Autodesk Inventor part; units mm, degrees
ref_plane "YZ Plane" through (0, 0, 0) normal (1, 0, 0) x (0, 1, 0)
ref_plane "XZ Plane" through (0, 0, 0) normal (0, 1, 0) x (-1, 0, 0)
ref_plane "XY Plane" through (0, 0, 0) normal (0, 0, 1) x (1, 0, 0)
sketch "Boceto1" plane through (0, 0, 0) normal (0, 0, 1) x (1, 0, 0)
  line L0 (206, -30) -> (206, 220)
  line L1 (0, 220) -> (206, 220)
  line L2 (0, -30) -> (0, 220)
  line L3 (206, -30) -> (0, -30)
  line L4 (206, -30) -> (206, -5)
  line L5 (206, -5) -> (203, -5)
  line L6 (203, -5) -> (203, 20)
  line L7 (203, 20) -> (206, 20)
  line L8 (206, 20) -> (206, 45)
  line L9 (206, 45) -> (203, 45)
  line L10 (203, 45) -> (203, 70)
  line L11 (203, 70) -> (206, 70)
  line L12 (206, 70) -> (206, 95)
  line L13 (206, 95) -> (203, 95)
  line L14 (203, 95) -> (203, 120)
  line L15 (203, 120) -> (206, 120)
  line L16 (206, 120) -> (206, 145)
  line L17 (206, 145) -> (203, 145)
  line L18 (203, 145) -> (203, 170)
  line L19 (203, 170) -> (206, 170)
  line L20 (203, 220) -> (206, 220)
  line L21 (206, 195) -> (203, 195)
  line L22 (203, 195) -> (203, 220)
  line L23 (206, 170) -> (206, 195)
  line L24 (203, 170) -> (206, 170)
  line L25 (0, 220) -> (0, 195)
  line L26 (0, 195) -> (3, 195)
  line L27 (3, 195) -> (3, 170)
  line L28 (3, 170) -> (0, 170)
  line L29 (0, 170) -> (0, 145)
  line L30 (0, 145) -> (3, 145)
  line L31 (3, 145) -> (3, 120)
  line L32 (3, 120) -> (0, 120)
  line L33 (3, 20) -> (0, 20)
  line L34 (0, 45) -> (3, 45)
  line L35 (3, 45) -> (3, 20)
  line L36 (0, 70) -> (0, 45)
  line L37 (3, 70) -> (0, 70)
  line L38 (3, 95) -> (3, 70)
  line L39 (0, 95) -> (3, 95)
  line L40 (0, 120) -> (0, 95)
  line L41 (3, 20) -> (0, 20)
  line L42 (0, 20) -> (0, -5)
  line L43 (0, -5) -> (3, -5)
  line L44 (3, -5) -> (3, -30)
  line L45 (3, -30) -> (0, -30)
  line L46 (203, 220) -> (206, 220)
  line L47 (203, 220) -> (206, 220)
  line L48 (206, 220) -> (206, 245)
  line L49 (206, 245) -> (203, 245)
  line L50 (203, 245) -> (203, 270)
  line L51 (203, 270) -> (206, 270)
  line L52 (0, 220) -> (3, 220)
  line L53 (0, 220) -> (3, 220)
  line L54 (3, 220) -> (3, 245)
  line L55 (3, 245) -> (0, 245)
  line L56 (0, 245) -> (0, 270)
  line L57 (0, 270) -> (3, 270)
  line L58 (206, 270) -> (0, 270)
  point P0 (0, 0)
  dimension "d78" = 3
  dimension "d88" = 3
  dimension "Lengueta" = 25
  dimension "espesor" = 3
  dimension "d2" = 25
  dimension "d3" = 3
  dimension "d4" = 25
  dimension "d5" = 90
  dimension "d6" = 3
  dimension "d7" = 25
  dimension "d8" = 3
  dimension "d9" = 25
  dimension "d10" = 3
  dimension "d11" = 25
  dimension "d12" = 3
  dimension "d13" = 25
  dimension "d14" = 90
  dimension "d15" = 3
  dimension "d16" = 25
  dimension "d17" = 3
  dimension "d18" = 3
  dimension "d19" = 25
  dimension "d20" = 90
  dimension "d21" = 3
  dimension "d22" = 25
  dimension "d23" = 3
  dimension "d26" = 25
  dimension "d27" = 3
  dimension "d28" = 25
  dimension "d29" = 3
  dimension "d30" = 25
  dimension "d31" = 90
  dimension "d32" = 3
  dimension "d33" = 25
  dimension "d34" = 3
  dimension "d35" = 25
  dimension "d36" = 3
  dimension "d37" = 25
  dimension "d38" = 3
  dimension "d39" = 25
  dimension "d40" = 90
  dimension "d41" = 3
  dimension "d42" = 25
  dimension "d43" = 3
  dimension "d44" = 3
  dimension "d45" = 25
  dimension "d46" = 90
  dimension "d47" = 3
  dimension "d48" = 25
  dimension "d49" = 3
  dimension "d71" = 3
  dimension "d72" = 3
  dimension "d73" = 25
  dimension "d74" = 90
  dimension "d75" = 3
  dimension "d76" = 25
  dimension "d77" = 3
  dimension "d81" = 3
  dimension "d82" = 3
  dimension "d83" = 25
  dimension "d84" = 90
  dimension "d85" = 3
  dimension "d86" = 25
  dimension "d87" = 3
extrude "Extrusión1" add sketch "Boceto1" against normal blind 3 contours L3 L44 L43 L2 L33 L35 L34 L37 L38 L39 L32 L31 L30 L28 L27 L26 L1 L22 L21 L0 L19 L18 L17 L15 L14 L13 L11 L10 L9 L7 L6 L5
sketch "Boceto2" plane through (0, 0, 0) normal (0, 0, 1) x (1, 0, 0)
  circle A0 centre (53, -15) radius 1.75
  circle A1 centre (153, -15) radius 1.75
  point P0 (0, 0)
extrude "Extrusión2" cut sketch "Boceto2" against normal blind 3
sketch "Boceto3" plane through (0, 0, 0) normal (0, 0, 1) x (1, 0, 0)
  circle A0 centre (53, 208) radius 2.1
  circle A1 centre (53, 208) radius 1.5
  circle A2 centre (153, 208) radius 2.1
  point P0 (0, 0)
  dimension "d56" = 3
hole "Agujero1" at (53, 208, 0) at (153, 208, 0) direction (0, 0, -1) diameter 3 depth 4
sketch "Boceto4" plane through (0, 0, 0) normal (0, 0, 1) x (1, 0, 0)
  circle A0 centre (53, 85) radius 2.1
  circle A1 centre (153, 85) radius 2.1
  point P0 (0, 0)
hole "Agujero2" at (153, 85, 0) at (53, 85, 0) direction (0, 0, -1) diameter 3 depth 4
sketch "Boceto5" plane through (0, 0, -3) normal (0, 0, -1) x (-1, 0, 0)
  point P0 (0, 0)
sketch "Boceto6" plane through (0, 0, 0) normal (0, 0, 1) x (1, 0, 0)
  circle A0 centre (53, 85) radius 1.5
  circle A1 centre (153, 85) radius 1.5
  circle A2 centre (153, 208) radius 1.5
  circle A3 centre (53, 208) radius 1.5
  circle A4 centre (53, -15) radius 1.75
  circle A5 centre (153, -15) radius 1.75
  line L0 (203, 20) -> (206, 20)
  line L1 (206, 20) -> (206, 45)
  line L2 (206, 45) -> (203, 45)
  line L3 (203, 45) -> (203, 70)
  line L4 (203, 70) -> (206, 70)
  line L5 (206, 70) -> (206, 95)
  line L6 (206, 95) -> (203, 95)
  line L7 (203, 95) -> (203, 120)
  line L8 (203, 120) -> (206, 120)
  line L9 (206, 120) -> (206, 145)
  line L10 (206, 145) -> (203, 145)
  line L11 (203, 145) -> (203, 170)
  line L12 (203, 170) -> (206, 170)
  line L13 (206, 170) -> (206, 195)
  line L14 (206, 195) -> (203, 195)
  line L15 (203, 195) -> (203, 220)
  line L16 (203, 220) -> (0, 220)
  line L17 (0, 220) -> (0, 195)
  line L18 (0, 195) -> (3, 195)
  line L19 (3, 195) -> (3, 170)
  line L20 (3, 170) -> (0, 170)
  line L21 (0, 170) -> (0, 145)
  line L22 (0, 145) -> (3, 145)
  line L23 (3, 145) -> (3, 120)
  line L24 (3, 120) -> (0, 120)
  line L25 (0, 120) -> (0, 95)
  line L26 (0, 95) -> (3, 95)
  line L27 (3, 95) -> (3, 70)
  line L28 (3, 70) -> (0, 70)
  line L29 (0, 70) -> (0, 45)
  line L30 (0, 45) -> (3, 45)
  line L31 (3, 45) -> (3, 20)
  line L32 (3, 20) -> (0, 20)
  line L33 (0, 20) -> (0, -5)
  line L34 (0, -5) -> (3, -5)
  line L35 (3, -5) -> (3, -30)
  line L36 (3, -30) -> (206, -30)
  line L37 (206, -30) -> (206, -5)
  line L38 (206, -5) -> (203, -5)
  line L39 (203, -5) -> (203, 20)
  line L40 (153, 85) -> (153, 208)
  line L41 (150.5, 161.5) -> (155.5, 161.5)
  line L42 (155.5, 161.5) -> (155.5, 131.5)
  line L43 (155.5, 131.5) -> (150.5, 131.5)
  line L44 (150.5, 131.5) -> (150.5, 161.5)
  line L45 (150.5, 161.5) -> (155.5, 131.5) construction
  line L46 (155.5, 161.5) -> (150.5, 131.5) construction
  line L47 (53, 85) -> (53, 208)
  line L48 (50.5, 161.5) -> (55.5, 161.5)
  line L49 (55.5, 161.5) -> (55.5, 131.5)
  line L50 (55.5, 131.5) -> (50.5, 131.5)
  line L51 (50.5, 131.5) -> (50.5, 161.5)
  line L52 (50.5, 161.5) -> (55.5, 131.5) construction
  line L53 (55.5, 161.5) -> (50.5, 131.5) construction
  line L54 (53, -15) -> (53, 85)
  line L55 (50.5, 50) -> (55.5, 50)
  line L56 (55.5, 50) -> (55.5, 20)
  line L57 (55.5, 20) -> (50.5, 20)
  line L58 (50.5, 20) -> (50.5, 50)
  line L59 (50.5, 50) -> (55.5, 20) construction
  line L60 (55.5, 50) -> (50.5, 20) construction
  line L61 (150.5, 50) -> (155.5, 50)
  line L62 (155.5, 50) -> (155.5, 20)
  line L63 (155.5, 20) -> (150.5, 20)
  line L64 (150.5, 20) -> (150.5, 50)
  line L65 (150.5, 50) -> (155.5, 20) construction
  line L66 (155.5, 50) -> (150.5, 20) construction
  point P0 (0, 0)
  point P1 (153, 146.5)
  point P2 (53, 146.5)
  point P3 (53, 35)
  point P4 (153, 35)
  dimension "d93" = 5
  dimension "d94" = 30
  dimension "d95" = 5
  dimension "d96" = 30
  dimension "d99" = 5
  dimension "d100" = 30
  dimension "d101" = 5
  dimension "d102" = 30
extrude "Extrusión3" cut sketch "Boceto6" against normal blind 3 contours L55 L56 L57 L54 | L54 L57 L58 L55 | L50 L51 L48 L47 | L47 L48 L49 L50 | L43 L44 L41 L40 | L40 L41 L42 L43 | L61 L62 L63 L64
sketch "Boceto7" plane through (0, 0, 0) normal (0, 0, 1) x (1, 0, 0)
  line L0 (3, 95.5) -> (60.5, 95.5)
  line L1 (60.5, 95.5) -> (60.5, 98.5)
  line L2 (60.5, 98.5) -> (3, 98.5)
  line L3 (3, 98.5) -> (3, 121)
  line L4 (3, 121) -> (60.5, 121)
  line L5 (60.5, 121) -> (60.5, 124)
  line L6 (60.5, 124) -> (3, 124)
  line L7 (3, 124) -> (3, 128)
  arc A0 (10.873, 129) -> (3, 128) centre (7, 128) ccw
  arc A1 (10.873, 129) -> (14.746, 126) centre (14.746, 130) ccw
  line L8 (14.746, 126) -> (57.754, 126)
  arc A2 (57.754, 126) -> (61.627, 129) centre (57.754, 130) ccw
  arc A3 (69.5, 128) -> (61.627, 129) centre (65.5, 128) ccw
  line L9 (69.5, 128) -> (69.5, 91.5)
  arc A4 (61.627, 90.5) -> (69.5, 91.5) centre (65.5, 91.5) ccw
  arc A5 (61.627, 90.5) -> (57.754, 93.5) centre (57.754, 89.5) ccw
  line L10 (57.754, 93.5) -> (14.746, 93.5)
  arc A6 (14.746, 93.5) -> (10.873, 90.5) centre (14.746, 89.5) ccw
  arc A7 (3, 91.5) -> (10.873, 90.5) centre (7, 91.5) ccw
  line L11 (3, 91.5) -> (3, 95.5)
  line L12 (66.1403, 93.5) -> (64.8597, 93.5)
  arc A8 (64.8597, 93.5) -> (66.1403, 93.5) centre (65.5, 91.5) ccw
  arc A9 (66.1403, 126) -> (64.8597, 126) centre (65.5, 128) ccw
  line L13 (64.8597, 126) -> (66.1403, 126)
  line L14 (6.3597, 126) -> (7.6403, 126)
  arc A10 (7.6403, 126) -> (6.3597, 126) centre (7, 128) ccw
  arc A11 (6.3597, 93.5) -> (7.6403, 93.5) centre (7, 91.5) ccw
  line L15 (7.6403, 93.5) -> (6.3597, 93.5)
  circle A12 centre (74.05, 124.85) radius 1.55
  circle A13 centre (90.35, 93.75) radius 1.55
  line L16 (92.9, 87.6) -> (71.5, 87.6)
  line L17 (71.5, 87.6) -> (71.5, 131)
  line L18 (71.5, 131) -> (92.9, 131)
  line L19 (92.9, 131) -> (92.9, 87.6)
  point P0 (0, 0)
hole "Agujero3" at (65.5, 128, 0) at (7, 128, 0) at (7, 91.5, 0) at (65.5, 91.5, 0) at (90.35, 93.75, 0) at (74.05, 124.85, 0) direction (0, 0, -1) diameter 3.1 end through all
sketch "Boceto8" plane through (0, 0, 0) normal (0, 0, 1) x (1, 0, 0)
  line L0 (0, 220) -> (203, 220)
  line L1 (0, 220) -> (3, 220)
  line L2 (3, 220) -> (18, 220)
  line L3 (18, 220) -> (18, 205)
  line L4 (18, 205) -> (3, 205)
  line L5 (3, 205) -> (3, 220)
  line L6 (16.3, 206.7) -> (16.3, 218.3)
  line L7 (16.3, 218.3) -> (4.7, 218.3)
  line L8 (4.7, 218.3) -> (4.7, 206.7)
  line L9 (4.7, 206.7) -> (16.3, 206.7)
  circle A0 centre (10.5, 218.3) radius 1.7
  line L10 (12.2, 218.3) -> (12.2, 220)
  line L11 (8.8, 218.3) -> (8.8, 220)
  point P0 (0, 0)
  dimension "d115" = 3
  dimension "d116" = 15
  dimension "d117" = 15
  dimension "d118" = 1.7
  dimension "d119" = 3.4
extrude "Extrusión4" cut sketch "Boceto8" against normal blind 10 contours L0 A0 L11 | L0 L10 A0 | A0 L7 | L7 A0
equation "\"d2\" = Lengueta"
equation "\"d3\" = espesor"
equation "\"d4\" = Lengueta"
equation "\"d6\" = espesor"
equation "\"d7\" = Lengueta"
equation "\"d8\" = espesor"
equation "\"d11\" = d9"
equation "\"d12\" = d10"
equation "\"d13\" = d9"
equation "\"d16\" = d9"
equation "\"d18\" = d24"
equation "\"d19\" = d25"
equation "\"d22\" = d25"
equation "\"d28\" = d26"
equation "\"d29\" = d27"
equation "\"d30\" = d26"
equation "\"d33\" = d26"
equation "\"d37\" = d35"
equation "\"d38\" = d36"
equation "\"d39\" = d35"
equation "\"d42\" = d35"
equation "\"d44\" = d50"
equation "\"d45\" = d51"
equation "\"d48\" = d51"
equation "\"d71\" = d78"
equation "\"d72\" = d79"
equation "\"d73\" = d80"
equation "\"d76\" = d80"
equation "\"d81\" = d88"
equation "\"d82\" = d89"
equation "\"d83\" = d90"
equation "\"d86\" = d90"
equation "\"d52\" = espesor"
equation "\"d54\" = espesor"
properties part number "Envolvente_Pared_Trasera"
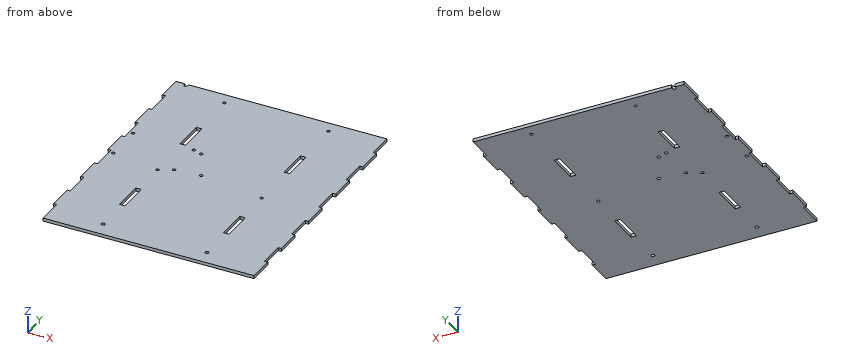
Source: CAD feature listing. Evaluate the final solid. Frame: model axes, mm. Round coordinates to 2 decimals unless told otherwise and drop trailing zeros. Use CSV: the item, a comma, the result in double quotes. Start each with the question number.
(1) First-contact query: pin 1 Ø0.9 at (y, z) = (34, -2) entering from -X; pin 2 Ø5 at (x, y) = (53, 85) entering from +Z. Flat tips, straight axial feed; report the tip coordinate or a pass-through.
(2) Material intervals for probe 1 along Y at (x, z) = (153, -1.4); probe 2 along X at (y, z) = (135, -2.8); probe 3 along X at (y, z) = (91.5, -2.2), sorted ascending. Write a range as [from, to].
(3) Cut plane A-A, the plane z = -0.7. Give the number of separate pieces and of enclosed holes in the cut face, and give its area (3 significant figures).
Geometry says:
1,pin 1,"x = 3"
1,pin 2,"z = 0"
2,probe 1,"[-30, -16.75], [-13.25, 20], [50, 83.5], [86.5, 131.5], [161.5, 206.5], [209.5, 220]"
2,probe 2,"[3, 50.5], [55.5, 150.5], [155.5, 206]"
2,probe 3,"[3, 5.45], [8.55, 63.95], [67.05, 206]"
3,separate pieces,"1"
3,enclosed holes,"16"
3,area,"50,000 mm²"
